Verification items for the finished model (mm, model axes). Face numbers are marked on the shaded views. A direction names the side the tool comes from. Coordinates: 2 decimals unless noted, no trailing zeros. Order: outer loops, then holes, each group sorted by start corner. A loop starts at its lowest first (then second) coordinate and runs counter-clockwise, first axis right, second up. Notation, with made-up numbers: (-3, 14.5) -> (26, 14.5) arc R10 cw to (26, 22.5) -> close; hole circle Ø7 at (-35, 11.5). An arc over 180 degrees is marked (long way). Write item = value, one per line. Start each with the question number.
from build123d import *

# Parameters (mm, degrees)
F0_R         = 1.5875
F1_DEPTH     = 4
F3_DEPTH     = 21
F4_SIZE      = 0.508
F5_R         = 1.5875
F6_DEPTH     = 5
F7_R         = 1.5875
F8_DEPTH     = 5.0038
F9_SIZE      = 0.3175
F12_DEPTH    = 9
F17_D        = 2
F17_ON_F14_D = 2
F17_ON_F16_D = 2
F17_ON_F15_D = 2
F19_DEPTH    = 12.00658
F21_DEPTH    = 27.1145
F22_W        = 17.5895
F22_H        = 9.525
F22_H_2      = 12.7
F23_DEPTH    = 10.16
F25_R        = 1.5875
F26_DEPTH    = 1.7145
F24_R        = 1.5875
F27_DEPTH    = 1.7145


with BuildPart() as f1:
    # F0 (on Top) → F1 (new body)
    with BuildSketch(Plane.XY):
        with BuildLine():
            Line((37.30625, 15.08125), (-37.30625, 15.08125))
            ThreePointArc((-37.30625, 15.08125), (-39.5513140303, 14.1513140303), (-40.48125, 11.90625))
            Line((-40.48125, 11.90625), (-40.48125, -11.90625))
            ThreePointArc((-40.48125, -11.90625), (-39.5513140303, -14.1513140303), (-37.30625, -15.08125))
            Line((-37.30625, -15.08125), (37.30625, -15.08125))
            ThreePointArc((37.30625, -15.08125), (39.5513140303, -14.1513140303), (40.48125, -11.90625))
            Line((40.48125, -11.90625), (40.48125, 11.90625))
            ThreePointArc((40.48125, 11.90625), (39.5513140303, 14.1513140303), (37.30625, 15.08125))
        make_face()
        with Locations((-35.48125, -9.08125)):
            Circle(F0_R, mode=Mode.SUBTRACT)
        with Locations((35.48125, -9.08125)):
            Circle(F0_R, mode=Mode.SUBTRACT)
        with Locations((-35.48125, 9.08125)):
            Circle(F0_R, mode=Mode.SUBTRACT)
        with BuildLine():
            ThreePointArc((-29.25, 9.90625), (-28.3200640303, 12.1513140303), (-26.075, 13.08125))
            Line((-26.075, 13.08125), (26.075, 13.08125))
            ThreePointArc((26.075, 13.08125), (28.3200640303, 12.1513140303), (29.25, 9.90625))
            Line((29.25, 9.90625), (29.25, -9.90625))
            ThreePointArc((29.25, -9.90625), (28.3200640303, -12.1513140303), (26.075, -13.08125))
            Line((26.075, -13.08125), (-26.075, -13.08125))
            ThreePointArc((-26.075, -13.08125), (-28.3200640303, -12.1513140303), (-29.25, -9.90625))
            Line((-29.25, -9.90625), (-29.25, 9.90625))
        make_face(mode=Mode.SUBTRACT)
        with Locations((35.48125, 9.08125)):
            Circle(F0_R, mode=Mode.SUBTRACT)
    extrude(amount=F1_DEPTH)

    # F2 (on face) → F3 (join)
    with BuildSketch(Plane.XY.offset(4)):
        with BuildLine():
            Line((28.075, 15.08125), (-28.075, 15.08125))
            ThreePointArc((-28.075, 15.08125), (-30.3200640303, 14.1513140303), (-31.25, 11.90625))
            Line((-31.25, 11.90625), (-31.25, -11.90625))
            ThreePointArc((-31.25, -11.90625), (-30.3200640303, -14.1513140303), (-28.075, -15.08125))
            Line((-28.075, -15.08125), (28.075, -15.08125))
            ThreePointArc((28.075, -15.08125), (30.3200640303, -14.1513140303), (31.25, -11.90625))
            Line((31.25, -11.90625), (31.25, 11.90625))
            ThreePointArc((31.25, 11.90625), (30.3200640303, 14.1513140303), (28.075, 15.08125))
        make_face()
        with BuildLine():
            ThreePointArc((-29.25, 9.90625), (-28.3200640303, 12.1513140303), (-26.075, 13.08125))
            Line((-26.075, 13.08125), (26.075, 13.08125))
            ThreePointArc((26.075, 13.08125), (28.3200640303, 12.1513140303), (29.25, 9.90625))
            Line((29.25, 9.90625), (29.25, -9.90625))
            ThreePointArc((29.25, -9.90625), (28.3200640303, -12.1513140303), (26.075, -13.08125))
            Line((26.075, -13.08125), (-26.075, -13.08125))
            ThreePointArc((-26.075, -13.08125), (-28.3200640303, -12.1513140303), (-29.25, -9.90625))
            Line((-29.25, -9.90625), (-29.25, 9.90625))
        make_face(mode=Mode.SUBTRACT)
    extrude(amount=F3_DEPTH)

    # F4
    f4_edges = [f1.edges().sort_by_distance(p)[0] for p in [
        (32.690625, -15.08125, 4),
        (39.551314, -14.151314, 4),
        (40.48125, 0, 4),
        (39.551314, 14.151314, 4),
        (32.690625, 15.08125, 4),
        (-32.690625, -15.08125, 4),
        (-39.551314, -14.151314, 4),
        (-40.48125, 0, 4),
        (-39.551314, 14.151314, 4),
        (-32.690625, 15.08125, 4),
    ]]
    chamfer(f4_edges, length=F4_SIZE)

    # F5 (on face) → F6 (join)
    with BuildSketch(Plane.YZ.offset(31.25)):
        with Locations((0, 18)):
            Circle(F5_R)
    extrude(amount=F6_DEPTH)

    # F7 (on face) → F8 (join)
    with BuildSketch(Plane(origin=(-31.25, 0, 0), x_dir=(0, -1, 0), z_dir=(-1, 0, 0))):
        with Locations((0, 17.9896)):
            Circle(F7_R)
    extrude(amount=F8_DEPTH)

    # F9
    f9_edges = [f1.edges().sort_by_distance(p)[0] for p in [
        (36.25, -1.5875, 18),
        (-36.2538, 1.5875, 17.9896),
    ]]
    chamfer(f9_edges, length=F9_SIZE)

    # F11 (on offset) → F12 (join)
    with BuildSketch(Plane.XY.offset(6.35)):
        with BuildLine():
            Line((-29.25, 13.08125), (-29.25, 7.08125))
            Line((-29.25, 7.08125), (-24.9645, 7.08125))
            ThreePointArc((-24.9645, 7.08125), (-23.7521654237, 7.5834154237), (-23.25, 8.79575))
            Line((-23.25, 8.79575), (-23.25, 13.08125))
            Line((-23.25, 13.08125), (-29.25, 13.08125))
        make_face()
        with BuildLine():
            ThreePointArc((-23.25, -8.79575), (-23.7521654237, -7.5834154237), (-24.9645, -7.08125))
            Line((-24.9645, -7.08125), (-29.25, -7.08125))
            Line((-29.25, -7.08125), (-29.25, -13.08125))
            Line((-29.25, -13.08125), (-23.25, -13.08125))
            Line((-23.25, -13.08125), (-23.25, -8.79575))
        make_face()
        with BuildLine():
            Line((29.25, -7.08125), (24.9645, -7.08125))
            ThreePointArc((24.9645, -7.08125), (23.7521654237, -7.5834154237), (23.25, -8.79575))
            Line((23.25, -8.79575), (23.25, -13.08125))
            Line((23.25, -13.08125), (29.25, -13.08125))
            Line((29.25, -13.08125), (29.25, -7.08125))
        make_face()
        with BuildLine():
            ThreePointArc((23.25, 8.79575), (23.7521654237, 7.5834154237), (24.9645, 7.08125))
            Line((24.9645, 7.08125), (29.25, 7.08125))
            Line((29.25, 7.08125), (29.25, 13.08125))
            Line((29.25, 13.08125), (23.25, 13.08125))
            Line((23.25, 13.08125), (23.25, 8.79575))
        make_face()
    extrude(amount=F12_DEPTH)

    # F17 (through all)
    with Locations(Plane.XY.offset(15.35)):
        with Locations((-26.075, 9.90625)):
            Hole(F17_D / 2)

    # F17 on F14 (through all)
    with Locations(Plane.XY.offset(15.35)):
        with Locations((-26.075, -9.90625)):
            Hole(F17_ON_F14_D / 2)

    # F17 on F16 (through all)
    with Locations(Plane.XY.offset(15.35)):
        with Locations((26.075, -9.90625)):
            Hole(F17_ON_F16_D / 2)

    # F17 on F15 (through all)
    with Locations(Plane.XY.offset(15.35)):
        with Locations((26.075, 9.90625)):
            Hole(F17_ON_F15_D / 2)

    # F18 (on face) → F19 (join)
    with BuildSketch(Plane(origin=(0, 15.08125, 0), x_dir=(-1, 0, 0), z_dir=(0, 1, 0))):
        with BuildLine():
            Line((-3.175, 4.5), (-13.49375, 4.5))
            Line((-13.49375, 4.5), (-13.49375, 1))
            Line((-13.49375, 1), (13.49375, 1))
            Line((13.49375, 1), (13.49375, 4.5))
            Line((13.49375, 4.5), (3.175, 4.5))
            ThreePointArc((3.175, 4.5), (0, 7.675), (-3.175, 4.5))
        make_face()
    extrude(amount=F19_DEPTH)

    # F20 (on face) → F21 (join)
    with BuildSketch(Plane.YZ.offset(13.49375)):
        Polygon((21.43125, 7.35), (21.43125, 1), (27.08783, 1), (31.4984937127, 26.0141169265), (25.0925369558, 30.7010801522), (21.9182232609, 30.7670920161), align=None)
    extrude(amount=-F21_DEPTH)

    # F22 (on face) → F23 (cut)
    with BuildSketch(Plane(origin=(0, 26.1000219104, -4.6021380599), x_dir=(-1, 0, 0), z_dir=(0, 0.984807753, -0.1736481777))):
        with Locations((0.0635, 12.1655600695)):
            Rectangle(F22_W, F22_H)
        with Locations((0.0635, 30.7710600695)):
            Rectangle(F22_W, F22_H_2)
    extrude(amount=-F23_DEPTH, mode=Mode.SUBTRACT)

    # F25 (on face) → F26 (cut)
    with BuildSketch(Plane(origin=(8.73125, 0, 0), x_dir=(0, -1, 0), z_dir=(-1, 0, 0))):
        with Locations((-24.9453486986, 23.623235759)):
            Circle(F25_R)
    extrude(amount=-F26_DEPTH, mode=Mode.SUBTRACT)

    # F24 (on face) → F27 (cut)
    with BuildSketch(Plane.YZ.offset(-8.85825)):
        with Locations((24.9363394923, 23.1900098967)):
            Circle(F24_R)
    extrude(amount=-F27_DEPTH, mode=Mode.SUBTRACT)


solid = f1.part
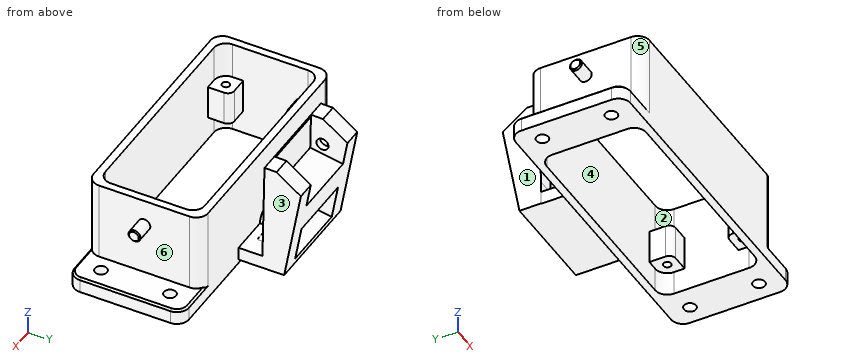
Item 1: Tool access check on the marked faces 1, 2 and 3. Record the directions out of +Z, -Z, +X, -X, +Y, -Y that give a thin tool (end or side, any length) a straight path to the whole face; none if there is none.
Item 2: Gauge pin test, flat ends, axial feed: P1, Ø10, axis at x = 29, z = 15, coming from the -Y side; P2, Ø9.5, axis at x = 1.5, y = 22, coming from the -Z side; P3, Ø6.5, axis at x = 26.5, y = -9, coming from the +Z side; P4, Ø6.5, axis at y = -3.5, z = 11.5, coming from the -X side. Record the tip position at first contact, or that the pin passes through.
Item 3: Section check A-A (x = 0). Record the boundary of the cut face in (y, z) (3 decimals).
Item 4: Thickness scan on line 1 (Y direction, x = -12.5, z = 21.5); line 2 (Y direction, x = 5, z = 21.5); line 3 (X direction, y = -2, z = 10.5). Record the ranges inside material, lowest first.
Item 5: Section check C-C (x = 12.5). Record the boundary of the cut face in (y, z).
Item 6: Section check D-D (z = 10). State how many separate pieces and enclosed holes the cut face has, then the cut area to 3 significant figures.
Item 7: Section check B-B (y = 0). Record the boundary of the cut face in (x, z).
Item 8: Mould release check, pull along Y, two halves, no side actions. Record for the marked faces 4, 5 and 6: pulls with the +Y half, pulls with the -Y half, needs draft (parallel to the pull), parting line crosses it, or undercut.
Filled sheet:
q1.face_1 = +Z, -Z, -X, +Y
q1.face_2 = +Z
q1.face_3 = +Z, -Z, +X, +Y
q2.P1 = -15.08
q2.P2 = 1
q2.P3 = 25
q2.P4 = -31.25
q3.outline = (-15.081, 0) -> (-13.081, 0) -> (-13.081, 25) -> (-15.081, 25) -> close; (13.081, 0) -> (15.081, 0) -> (15.081, 1) -> (27.088, 1) -> (27.386, 2.688) -> (17.38, 4.453) -> (17.948, 7.675) -> (15.081, 7.675) -> (15.081, 25) -> (13.081, 25) -> close; (21.557, 13.388) -> (29.04, 12.069) -> (30.341, 19.448) -> (21.714, 20.969) -> close; (21.905, 30.114) -> (22.019, 30.765) -> (21.918, 30.767) -> close
q4.line_1 = -15.08 to -13.08, 13.08 to 15.08, 21.73 to 30.7
q4.line_2 = -15.08 to -13.08, 13.08 to 15.08
q4.line_3 = -31.25 to -29.25, 29.25 to 31.25
q5.outline = (-15.08, 0) -> (-13.08, 0) -> (-13.08, 25) -> (-15.08, 25) -> close; (13.08, 0) -> (15.08, 0) -> (15.08, 1) -> (27.09, 1) -> (31.5, 26.01) -> (25.09, 30.7) -> (21.92, 30.77) -> (21.43, 7.35) -> (21.43, 4.5) -> (15.08, 4.5) -> (15.08, 25) -> (13.08, 25) -> close
q6.separate_pieces = 3
q6.enclosed_holes = 5
q6.area = 543 mm^2
q7.outline = (-40.48, 0) -> (-29.25, 0) -> (-29.25, 25) -> (-31.25, 25) -> (-31.25, 19.58) -> (-35.94, 19.58) -> (-36.25, 19.26) -> (-36.25, 16.72) -> (-35.94, 16.4) -> (-31.25, 16.4) -> (-31.25, 4) -> (-39.97, 4) -> (-40.48, 3.49) -> close; (29.25, 0) -> (40.48, 0) -> (40.48, 3.49) -> (39.97, 4) -> (31.25, 4) -> (31.25, 16.41) -> (35.93, 16.41) -> (36.25, 16.73) -> (36.25, 19.27) -> (35.93, 19.59) -> (31.25, 19.59) -> (31.25, 25) -> (29.25, 25) -> close
q8.face_4 = undercut
q8.face_5 = pulls with the -Y half
q8.face_6 = needs draft
